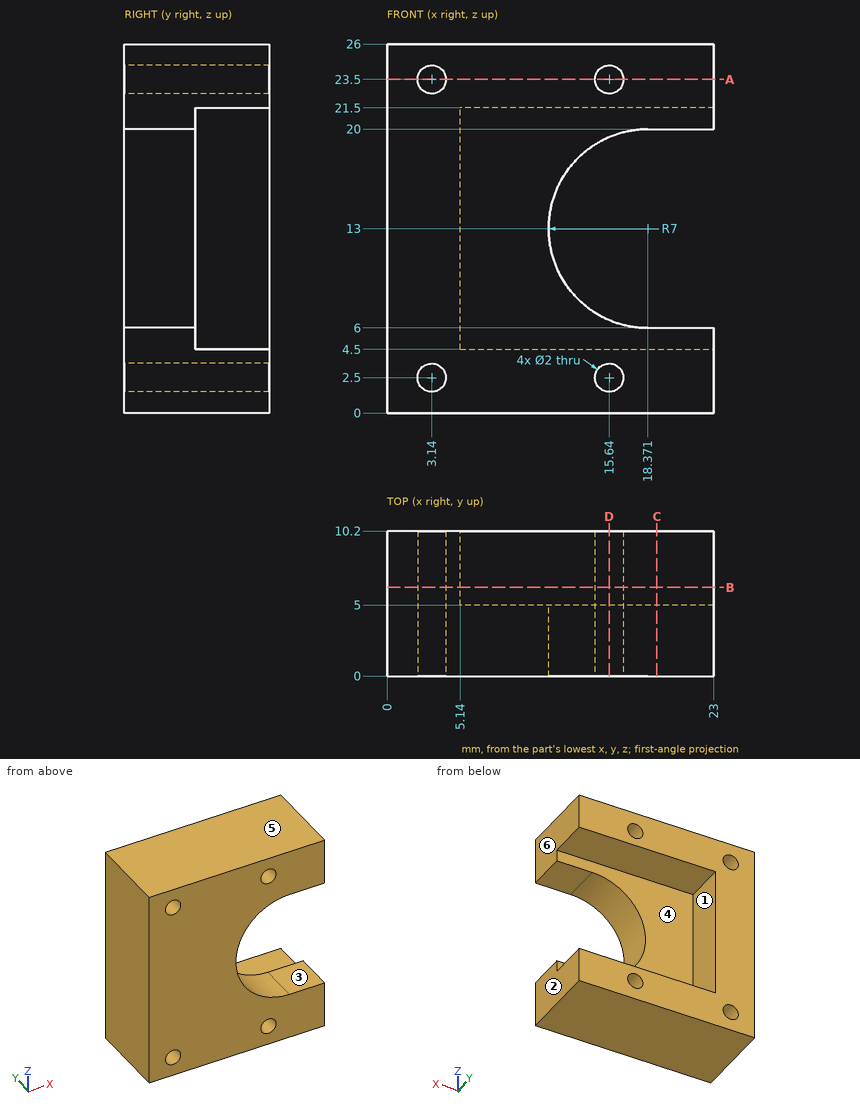
Here's the drawing with two shaded views (mm, measured from the low corner). I have some questions. A direction names the side the tool comes from. Coordinates: 2 decimals unless noted, no trailing zeros. Order: outer loops, then holes, each group sorted by start corner. A loop starts at its lowest first (then second) coordinate and runs counter-clockwise, first axis right, second up. Notation, with made-up numbers: M -17.5,-32 L 4.5,-32 A20 cw 4.5,-26 Z; hole C 19,86.25 d6. An arc over 180 degrees is marked long. Write item = value, one per line.
(1) Suppose I cut it at A-A on z = 23.5. Please give me the cut outline in (x, y), plus the area to 3 significant figures.
Results are:
outline = M 0,0 L 2.14,0 L 2.14,10.2 L 0,10.2 Z; M 4.14,0 L 14.64,0 L 14.64,10.2 L 4.14,10.2 Z; M 16.64,0 L 23,0 L 23,10.2 L 16.64,10.2 Z
area = 194 mm2
(2) Suppose I cut it at C-C on x = 19. Please give me the cut outline in (y, z).
Results are:
outline = M 0,0 L 10.2,0 L 10.2,4.5 L 5,4.5 L 5,6 L 0,6 Z; M 0,20 L 5,20 L 5,21.5 L 10.2,21.5 L 10.2,26 L 0,26 Z
(3) Suppose I cut it at D-D on x = 15.64. Please give me the cut outline in (y, z) (1 decimal).
Results are:
outline = M 0,0 L 10.2,0 L 10.2,1.5 L 0,1.5 Z; M 0,3.5 L 10.2,3.5 L 10.2,4.5 L 5,4.5 L 5,6.6 L 0,6.6 Z; M 0,19.4 L 5,19.4 L 5,21.5 L 10.2,21.5 L 10.2,22.5 L 0,22.5 Z; M 0,24.5 L 10.2,24.5 L 10.2,26 L 0,26 Z
(4) I need wall thicknesses on line 1 along Z through (x, y) = (3.14, 3); line 2 along Z through (x, y) = (15.64, 7.5); line 3 along Z through (x, y) = (13.5, 6.5). Which ranges of each line are inside material? Lowest first, please. Write a range as [from, to].
Results are:
line_1 = [0, 1.5], [3.5, 22.5], [24.5, 26]
line_2 = [0, 1.5], [3.5, 4.5], [21.5, 22.5], [24.5, 26]
line_3 = [0, 4.5], [21.5, 26]
(5) For pin 1 Ø3 at (y, z) = (2, 11.5) entering from +X; pin 2 Ø3 at (y, z) = (5, 16.5) entering from +X; pin 3 Ø5.5 at (y, z) = (8.5, 15) entering from +X, each with a flat end and sliding along its axis, tell me the tip position at first contact or that it passes through.
Results are:
pin_1 = 12.05
pin_2 = 13.47
pin_3 = 5.14
(6) For the marked faces 1, 2 and 3, which set-ups out of +Z, -Z, +X, -X, +Y, -Y let a thin tool reach every point of the face, with its end or its side?
Results are:
face_1 = +X, +Y
face_2 = +Z, -Z, +X, +Y, -Y
face_3 = +X, +Y, -Y
(7) If we mould it in two halves opening along Z, with no side actions, what happens to the marked faces 4, 5 and 6? For each: pulls with the +Z half, pulls with the -Z half, needs draft (parallel to the pull), parting line crosses it, or undercut.
Results are:
face_4 = undercut
face_5 = pulls with the +Z half
face_6 = needs draft
(8) Suppose I cut it at B-B on y = 6.25. Please give me the cut outline in (x, z), plus the area to 3 significant figures.
Results are:
outline = M 0,0 L 23,0 L 23,4.5 L 5.14,4.5 L 5.14,21.5 L 23,21.5 L 23,26 L 0,26 Z; hole C 3.14,2.5 d2; hole C 3.14,23.5 d2; hole C 15.64,2.5 d2; hole C 15.64,23.5 d2
area = 282 mm2
